The figure shows three views and two pictorial views of one solid part (mm, origin at its lowest corner). Answer the questions. Round coordinates to 2 decimals unless told otherwise and drop trailing zeros. Order: outer loops, then holes, each group sorted by start corner. A loop starts at its lowest first (then second) coordinate and runs counter-clockwise, first axis right, second up. Notation, with made-up numbers: (-0.5, 66.5) - (32.5, 66.5) arc R6 cw to (32.5, 75.5) - close; hole circle Ø2 at (21, 80.25). An arc over 180 degrees is marked (long way). Answer in a Markdown table with one row per item.
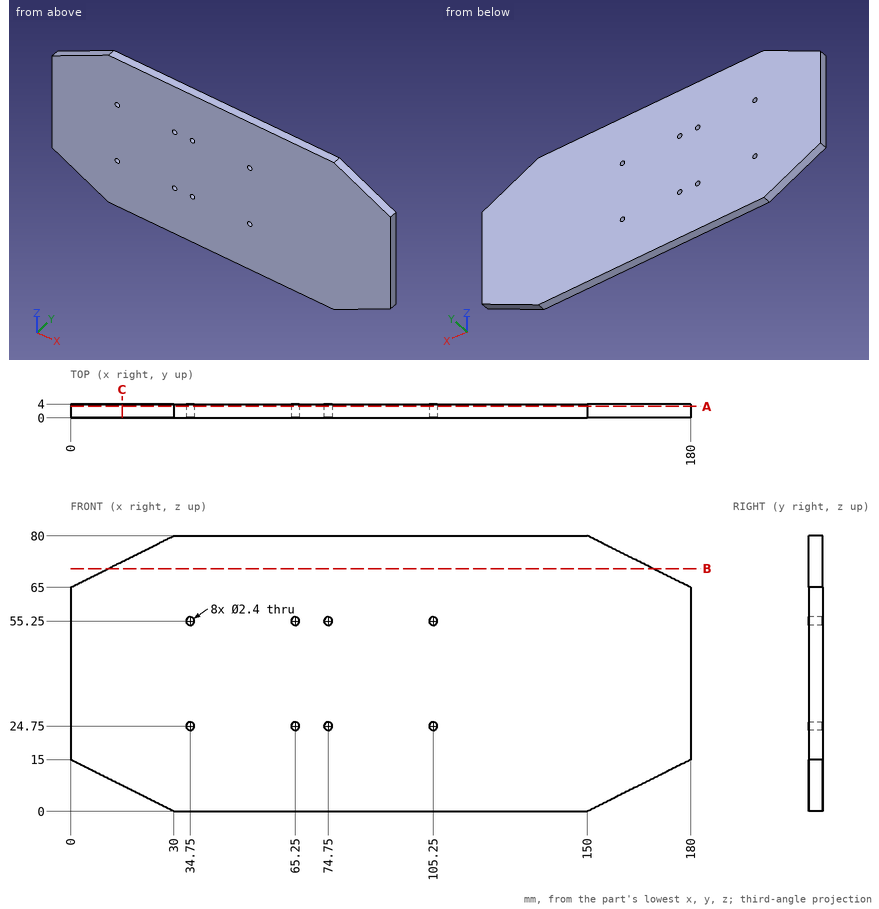
1) Find section A-A, the plane y = 3.3. Give the number of separate pieces and of enclosed holes in the cut face, then the cut area to 3 significant figures.
Filled in:
| item | result |
|---|---|
| separate pieces | 1 |
| enclosed holes | 8 |
| area | 13,500 mm^2 |
2) Find section B-B, the plane z = 70.5. Give the vertices of the cut face in (x, y).
Filled in:
| item | result |
|---|---|
| outline | (11, 0) - (169, 0) - (169, 4) - (11, 4) - close |
3) Find the intervals of material crossed by probe 1 along X at (y, z) = (1.5, 55); probe 2 along Z at (x, y) = (74.75, 2.5); probe 3 along Z at (x, y) = (161.5, 2.8), in increasing order. Write a range as from..to.
Filled in:
| item | result |
|---|---|
| probe 1 | x = 0..33.58, 35.92..64.08, 66.42..73.58, 75.92..104.08, 106.42..180 |
| probe 2 | z = 0..23.55, 25.95..54.05, 56.45..80 |
| probe 3 | z = 5.75..74.25 |
4) This flat-tipped pin is pushed along its axis until it touches: pin 1 (1 mm diameter, centred on y = 3, z = 69, fed in from +X). Where does it stop, or does it pass through?
Filled in:
| item | result |
|---|---|
| pin 1 | stops at x = 173 |
5) Find section C-C, the plane x = 15. Give the vertices of the cut face in (y, z).
Filled in:
| item | result |
|---|---|
| outline | (0, 7.5) - (4, 7.5) - (4, 72.5) - (0, 72.5) - close |
